```python
from build123d import *

# Parameters (mm, degrees)
F0_R     = 15
F1_DEPTH = 2
F3_DEPTH = 2


with BuildPart() as f1:
    # F0 (on Top) → F1 (new body)
    with BuildSketch(Plane.XY):
        Circle(F0_R)
    extrude(amount=F1_DEPTH)

    # F2 (on face) → F3 (join)
    with BuildSketch(Plane.XY.offset(2)):
        with BuildLine():
            ThreePointArc((-11.658853, 6.935612), (-7.132737, 7.1853), (-2.649061, 6.518432))
            ThreePointArc((-2.649061, 6.518432), (-0.916188, 7.486954), (-1.790806, 9.269067))
            ThreePointArc((-1.790806, 9.269067), (-7.078127, 9.596414), (-11.658853, 6.935612))
        make_face()
        with BuildLine():
            ThreePointArc((2.752731, 6.455697), (2.882497, 8.058589), (2.909441, 9.6665))
            ThreePointArc((2.909441, 9.6665), (1.314728, 11.221448), (-0.248597, 9.634947))
            ThreePointArc((-0.248597, 9.634947), (-0.29574, 7.705033), (-0.45524, 5.781143))
            ThreePointArc((-0.45524, 5.781143), (-2.191095, 4.842409), (-3.684971, 3.552933))
            ThreePointArc((-3.684971, 3.552933), (-2.214478, 3.73532), (-0.735143, 3.820066))
            ThreePointArc((-0.735143, 3.820066), (-3.092594, -3.950169), (-7.269774, -10.913309))
            ThreePointArc((-7.269774, -10.913309), (-1.185509, -4.467947), (2.281617, 3.689258))
            ThreePointArc((2.281617, 3.689258), (3.812787, 3.465108), (5.324822, 3.135752))
            ThreePointArc((5.324822, 3.135752), (7.057695, 4.104274), (6.183076, 5.886387))
            ThreePointArc((6.183076, 5.886387), (4.495229, 6.335689), (2.752731, 6.455697))
        make_face()
        with BuildLine():
            ThreePointArc((0.704108, -14.295988), (8.282362, -5.237022), (10.883323, 6.28382))
            ThreePointArc((10.883323, 6.28382), (9.288611, 7.838769), (7.725285, 6.252267))
            ThreePointArc((7.725285, 6.252267), (5.946495, -4.613602), (0.704108, -14.295988))
        make_face()
    extrude(amount=F3_DEPTH)


solid = f1.part
```
Work out the finished part from the listing and answer in its coordinate system (mm). A direction names the side the tool comes from. Round coordinates to 2 decimals unless told otherwise and drop trailing zeros. Loops run counter-clockwise (first coordinate to the right, second up) from the corner with the lowest first, then second, coordinate; pieces in that order, holes last. Notation, with made-up numbers: (18.5, 18) -> (67.5, 18) arc R11 cw to (67.5, 37) -> close; hole circle Ø7 at (74, 78). An arc over 180 degrees is marked (long way). Write each question's results on one line, items separated by ' | '. Start each with the question number.
1. For a pull along X with two mould halves and no side action, classify faces 1 (the face through (-2.168, 4.858, 2.986)), 2 (the face through (0, 3, 4)), 3 (the face through (5.996, -4.467, 2.986)) as +X half, -X half, draft (parallel to the pull), parting line (faces both ways), or undercut.
2. Section C-C (z = 1.5) is taken. Determine the outline of the cut face in (x, y).
3. Section D-D (y = 0) is taken. Determine the outline of the cut face in (x, z), plus the area to 3 significant figures.
4. Section A-A (z = 3.4) is taken. Determine the outline of the cut face in (x, y) (1 decimal), plus the area to 3 significant figures.
5. A tool of negligible diameter and unlimited length cuts with its end or side. For faces 4 (the face through (0, 0, 0)), 5 (the face through (-7.005, 9.613, 2.986)), 6 (the face through (-0.926, 7.458, 2.986)), from which of +Z, -Z, +X, -X, +Y, -Y can it reach the whole face along a straight path? Write none if from no direction.
6. Find the intervals of material crossed by probe 1 along Y at (x, z) = (0.25, 1.5); probe 2 along Z at (x, y) = (2.75, -1.75); probe 3 along X at (y, z) = (3, 2.7), in increasing order. Write a range as from..to.
7. Given pin 1 Ø1.5 at (x, z) = (-7.5, 0.5) entering from +Y; pin 2 Ø2 at (y, z) = (-4, 2) entering from +X, each flat-ended and moving along its own axis, determine where each tip first touches the part or whether it passes through.
8. Section B-B (y = -5.5) is taken. Determine the outline of the cut face in (x, z), plus the area to 3 significant figures.
Evaluation:
1) face 1: -X half | face 2: draft | face 3: undercut
2) outline: circle Ø30 at (0, 0)
3) outline: (-15, 0) -> (15, 0) -> (15, 2) -> (10.18, 2) -> (10.18, 4) -> (7.16, 4) -> (7.16, 2) -> (1.13, 2) -> (1.13, 4) -> (-1.63, 4) -> (-1.63, 2) -> (-15, 2) -> close | area: 71.6 mm2
4) outline: (-11.7, 6.9) arc R22.4 cw to (-2.6, 6.5) arc R1.4 ccw to (-1.8, 9.3) arc R9.1 ccw to start; (-7.3, -10.9) arc R25.1 ccw to (2.3, 3.7) arc R22.4 cw to (5.3, 3.1) arc R1.4 ccw to (6.2, 5.9) arc R9.1 ccw to (2.8, 6.5) arc R25.1 ccw to (2.9, 9.7) arc R1.6 ccw to (-0.2, 9.6) arc R33.1 cw to (-0.5, 5.8) arc R9.1 ccw to (-3.7, 3.6) arc R22.4 cw to (-0.7, 3.8) arc R33.1 cw to start; (0.7, -14.3) arc R25.1 ccw to (10.9, 6.3) arc R1.6 ccw to (7.7, 6.3) arc R33.1 cw to start | area: 144 mm2
5) face 4: -Z, +X, -X, +Y, -Y | face 5: +Z, +Y | face 6: +Z
6) probe 1: y = -15..15 | probe 2: z = 0..2 | probe 3: x = -0.89..2.11, 7.58..10.72
7) pin 1: stops at y = 13.4 | pin 2: stops at x = 14.7
8) outline: (-13.96, 0) -> (13.96, 0) -> (13.96, 2) -> (8.15, 2) -> (8.15, 4) -> (5.63, 4) -> (5.63, 2) -> (-1.9, 2) -> (-1.9, 4) -> (-3.83, 4) -> (-3.83, 2) -> (-13.96, 2) -> close | area: 64.7 mm2
